from build123d import *

# Parameters (mm, degrees)
BOSS_EXTRU_1_DEPTH          = 48
ENL_V_MAT_EXTRU_1_REACH     = 67.843
BOSS_EXTRU_2_DEPTH          = 48
ESQUISSE3_R                 = 1.9
ESQUISSE3_W                 = 5
ESQUISSE3_H                 = 4
ESQUISSE3_W_2               = 4
ESQUISSE3_H_2               = 5
BOSS_EXTRU_3_DEPTH          = 6
SYM_TRIE3_COPY_1_SKETCH_R   = 1.9
SYM_TRIE3_COPY_1_SKETCH_W   = 5
SYM_TRIE3_COPY_1_SKETCH_H   = 4
SYM_TRIE3_COPY_1_SKETCH_W_2 = 4
SYM_TRIE3_COPY_1_SKETCH_H_2 = 5
SYM_TRIE3_COPY_1_DEPTH      = 6
ESQUISSE5_W                 = 20
ESQUISSE5_H                 = 5
ENL_V_MAT_EXTRU_2_DEPTH     = 7


with BuildPart() as part:
    # Esquisse1 → Boss.-Extru.1 (new body)
    with BuildSketch(Plane(origin=(0, 0, 0), x_dir=(1, 0, 0), z_dir=(0, 1, 0))):
        Polygon((-31.25, 0), (31.25, 0), (37.5, 10.825317547), (12.948729811, 25), (10, 25), (10, 5), (-10, 5), (-10, 25), (-12.948729811, 25), (-37.5, 10.825317547), align=None)
    extrude(amount=BOSS_EXTRU_1_DEPTH)

    # Esquisse2 → Enlèv. mat.-Extru.1 (cut, up to next)
    with BuildSketch(Plane(origin=(0, 48, 0), x_dir=(1, 0, 0), z_dir=(0, 1, 0)), mode=Mode.PRIVATE) as enl_v_mat_extru_1_sk1:
        Polygon((-36, 8.227241336), (-16, 19.77424672), (-13, 19.77424672), (-13, 0), (-31.25, 0), align=None)
    enl_v_mat_extru_1_tool1 = extrude(enl_v_mat_extru_1_sk1.sketch, amount=-ENL_V_MAT_EXTRU_1_REACH, mode=Mode.PRIVATE) & part.part
    enl_v_mat_extru_1 = enl_v_mat_extru_1_tool1.solids().sort_by_distance((-22.148909, 48, -8.14347))[0]
    add(enl_v_mat_extru_1, mode=Mode.SUBTRACT)

    # Symétrie1: Enlèv. mat.-Extru.1 across plane
    add(enl_v_mat_extru_1.mirror(Plane(origin=(0, 0, 0), x_dir=(0, 0, 1), z_dir=(1, 0, 0))), mode=Mode.SUBTRACT)

    # Esquisse4 → Boss.-Extru.2 (add)
    with BuildSketch(Plane(origin=(0, 0, 0), x_dir=(1, 0, 0), z_dir=(0, 1, 0))):
        Polygon((-37.5, 10.825317547), (-31.25, 0), (31.25, 0), (37.5, 10.825317547), (34.901923789, 12.325317547), (29.517949192, 3), (-29.517949192, 3), (-34.901923789, 12.325317547), align=None)
    extrude(amount=BOSS_EXTRU_2_DEPTH)

    # Esquisse3 → Boss.-Extru.3 (add)
    with BuildSketch(Plane(origin=(-14.0625, 0, -24.356964481), x_dir=(0.8660254037844396, 0, -0.4999999999999984), z_dir=(0.49999999999999833, 0, 0.8660254037844395))):
        with Locations((-14.063293868, 38)):
            Circle(ESQUISSE3_R)
        with Locations((-14.063293868, 46)):
            Rectangle(ESQUISSE3_W, ESQUISSE3_H)
        with Locations((-22.063293868, 38)):
            Rectangle(ESQUISSE3_W_2, ESQUISSE3_H_2)
        with Locations((-6.063293868, 38)):
            Rectangle(ESQUISSE3_W_2, ESQUISSE3_H_2)
        with Locations((-14.063293868, 30)):
            Rectangle(ESQUISSE3_W, ESQUISSE3_H)
    boss_extru_3 = extrude(amount=-BOSS_EXTRU_3_DEPTH)

    # Symétrie2: Boss.-Extru.3 across plane
    add(boss_extru_3.mirror(Plane.ZX.offset(24)))

    # Symétrie3: Boss.-Extru.3 across plane
    add(boss_extru_3.mirror(Plane(origin=(0, 0, 0), x_dir=(0, 0, 1), z_dir=(1, 0, 0))))

    # Symétrie3 copy 1 sketch → Symétrie3 copy 1 (add)
    with BuildSketch(Plane(origin=(14.0625, 48, -24.356964481), x_dir=(-0.8660254037844396, 0, -0.4999999999999984), z_dir=(-0.49999999999999833, 0, 0.8660254037844395))):
        with Locations((-14.063293868, 38)):
            Circle(SYM_TRIE3_COPY_1_SKETCH_R)
        with Locations((-14.063293868, 46)):
            Rectangle(SYM_TRIE3_COPY_1_SKETCH_W, SYM_TRIE3_COPY_1_SKETCH_H)
        with Locations((-22.063293868, 38)):
            Rectangle(SYM_TRIE3_COPY_1_SKETCH_W_2, SYM_TRIE3_COPY_1_SKETCH_H_2)
        with Locations((-6.063293868, 38)):
            Rectangle(SYM_TRIE3_COPY_1_SKETCH_W_2, SYM_TRIE3_COPY_1_SKETCH_H_2)
        with Locations((-14.063293868, 30)):
            Rectangle(SYM_TRIE3_COPY_1_SKETCH_W, SYM_TRIE3_COPY_1_SKETCH_H)
    extrude(amount=-SYM_TRIE3_COPY_1_DEPTH)

    # Esquisse5 → Enlèv. mat.-Extru.2 (cut)
    with BuildSketch(Plane(origin=(0, 0, 0), x_dir=(1, 0, 0), z_dir=(0, 1, 0))):
        with Locations((0, 2.5)):
            Rectangle(ESQUISSE5_W, ESQUISSE5_H)
    extrude(amount=ENL_V_MAT_EXTRU_2_DEPTH, mode=Mode.SUBTRACT)


solid = part.part
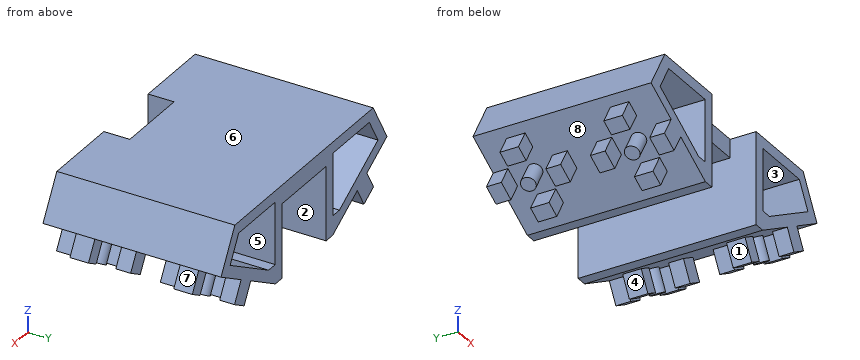
Model file for the job. Use its own axes, mm. Face numbers are marked on the shaded views. A direction names the side the tool comes from. Round coordinates to 2 decimals unless told otherwise and drop trailing zeros. Loops run counter-clockwise (first coordinate to the right, second up) from the corner with the lowest first, then second, coordinate; pieces in that order, holes last. Notation, with made-up numbers: (18, -23.75) -> (59, -23.75) arc R10 cw to (59, -8.75) -> close; hole circle Ø3 at (24.5, 20). An arc over 180 degrees is marked (long way). Answer as CSV lines item,"result". Start each with the question number.
1) Slice it at B-B (x = -23). List the corners of the cut face in (y, z), plus the area to 3 significant figures.
2) Slice it at D-D (x = 2.5). List the corners of the cut face in (y, z), plus the area to 3 significant figures.
3) Tool access for the marked faces 4, 5, 6, 7 and 8: list every direction of +Z, -Z, +X, -X, +Y, -Y with a clear straight run to the whole face (end or side of a thin tool).
4) Slice it at C-C (y = 25.5). List the corners of the cut face in (x, z), plus the area to 3 significant figures.
5) Probe line 1 along X through (y, z) = (34, -16.25); line 2 along Z through (x, y) = (-31, 19); line 3 along X through (y, z) = (35, -8.5). List the from-to ranges inside material, lowest first.
6) Pin check, flat tips, straight feed: P1, Ø4, axis at x = 30, z = -8.5, coming from the +Y side; P2, Ø1.9, axis at x = -22, z = -25.5, coming from the +Y side; P3, Ø5, axis at x = 3, y = 18.5, coming from the -Z side; P4, Ø3, axis at y = 39, z = -10, coming from the -X side. Stop position of each tip, or through.
7) Mould opens along Z. For the marked faces 1, 2 and 3 say: +Z half, -Z half, draft (parallel to the pull), parting line (faces both ways), or undercut.
8) Slice it at A-A (y = 18). List the corners of the cut face in (x, z).
Filled in:
1,outline,"(0, -19.2) -> (48, -19.2) -> (48, -15.73) -> (0, -15.73) -> close; (0, -3) -> (48, -3) -> (48, 0) -> (0, 0) -> close; (7.5, -26.13) -> (12.5, -26.13) -> (12.5, -23.71) -> (7.5, -23.71) -> close; (35.5, -26.13) -> (40.5, -26.13) -> (40.5, -23.71) -> (35.5, -23.71) -> close"
1,area,"334 mm2"
2,outline,"(7, -5) -> (48, -5) -> (48, 0) -> (7, 0) -> close"
2,area,"205 mm2"
3,face 4,"-Z, +Y, -Y"
3,face 5,"+Y, -Y"
3,face 6,"+Z, +X, -X, +Y, -Y"
3,face 7,"+X, +Y, -Y"
3,face 8,"none"
4,outline,"(-37.5, -10.83) -> (-12.95, -25) -> (-10, -25) -> (-10, -5) -> (10, -5) -> (10, -25) -> (12.95, -25) -> (37.5, -10.83) -> (31.25, 0) -> (-31.25, 0) -> close; hole (-33.4, -9.73) -> (-16, -19.77) -> (-13, -19.77) -> (-13, -3) -> (-29.52, -3) -> close; hole (13, -19.77) -> (16, -19.77) -> (33.4, -9.73) -> (29.52, -3) -> (13, -3) -> close"
4,area,"576 mm2"
5,line 1,"x = -28.1 to -22.1, -13 to -10, 10 to 13, 22.1 to 28.1"
5,line 2,"z = -21.51 to -20.57, -14.58 to -11.11, -5.57 to 0"
5,line 3,"x = -36.16 to -32.69, -13 to -10, 10 to 13, 32.69 to 36.16"
6,P1,"passes through"
6,P2,"stops at y = 40.5"
6,P3,"stops at z = -5"
6,P4,"stops at x = -37.5"
7,face 1,"-Z half"
7,face 2,"draft"
7,face 3,"undercut"
8,outline,"(-37.5, -10.83) -> (-28.41, -16.08) -> (-31.41, -21.27) -> (-27.08, -23.77) -> (-24.08, -18.58) -> (-12.95, -25) -> (-10, -25) -> (-10, -5) -> (10, -5) -> (10, -25) -> (12.95, -25) -> (24.08, -18.58) -> (27.08, -23.77) -> (31.41, -21.27) -> (28.41, -16.08) -> (37.5, -10.83) -> (31.25, 0) -> (-31.25, 0) -> close; hole (-33.4, -9.73) -> (-16, -19.77) -> (-13, -19.77) -> (-13, -3) -> (-29.52, -3) -> close; hole (13, -19.77) -> (16, -19.77) -> (33.4, -9.73) -> (29.52, -3) -> (13, -3) -> close"
